Geometry check sheet. Reference: the model listing, model coordinates, mm. A direction names the side the tool comes from. Coordinates: 2 decimals unless noted, no trailing zeros. Loops run counter-clockwise (first coordinate to the right, second up) from the corner with the lowest first, then second, coordinate; pieces in that order, holes last. Notation, with made-up numbers: (86.25, 65) - (90.25, 65) arc R31 cw to (90.25, 102) - close; hole circle Ø6 at (33.25, -32.75). An arc over 180 degrees is marked (long way). Write each question's results on one line, items separated by ' | '. Start each with the question number.
(1) Access from +Z, -Z, +X, -X, +Y, -Y to the whole of each face (thin tool, end or side, straight path). Record for faces 1 (the face through (45, 10, 30)), 2 (the face through (6, 12, 10)), 3 (the face through (31, 9.9, 48.2)), 4 (the face through (30.44, 9.86, 20.76)), 5 (the face through (30, 10, 0)).
(2) Sectioned sample at A-A (z = 31). Enter the section's corners in (x, y), plus the area to 3 significant figures.
(3) Sectioned sample at D-D (y = 18). Enter the section's corners in (x, z).
(4) Sectioned sample at B-B (x = 39). Enter the section's corners in (y, z), plus the area to 3 significant figures.
(5) Material ranges on probe 1 along X at (y, z) = (10, 4); probe 2 along X at (y, z) = (2.75, 41.5); probe 3 along X at (y, z) = (10.5, 3.5) (3 decimals), recorded low to high.
(6) Go/stop test with flat-tipped pins: pin 1 Ø2 at (y, z) = (7, 12) entering from -X; pin 2 Ø5.5 at (x, y) = (7.5, 10) entering from +Z; pin 3 Ø4 at (y, z) = (14.5, 16.5) entering from +X; pin 4 Ø12 at (x, y) = (9.5, 9) entering from +Z. Record where each tip stops, or that it passes through.
(7) Mould release check, pull along Z, two halves, no side actions. Record for faces 6 (the face through (22, 10, 51)), 7 (the face through (30, 0, 19)), 8 (the face through (21.902, 10.585, 43.405)): pulls with the +Z half, pulls with the -Z half, needs draft (parallel to the pull), parting line crosses it, or undercut.
(8) Sectioned sample at C-C (x = 7.5). Enter the section's corners in (y, z), plus the area to 3 significant figures.
from build123d import *

# Parameters (mm, degrees)
BOX002_W                    = 2
BOX002_H                    = 25
BOX002_DEPTH                = 15
CYLINDER003_R               = 2.3
CYLINDER003_DEPTH           = 33
CYLINDER003_PITCH_ANGLE     = 90
CYLINDER003_PLACEMENT_ANGLE = 7e-06
CYLINDER002_R               = 2.3
CYLINDER002_DEPTH           = 13
CYLINDER001_R               = 2.3
CYLINDER001_DEPTH           = 13
CYLINDER_R                  = 10.25
CYLINDER_DEPTH              = 25
CYLINDER_ROLL_ANGLE         = -90
BOX001_W                    = 30
BOX001_H                    = 20
BOX001_DEPTH                = 41
BOX_W                       = 60
BOX_H                       = 20
BOX_DEPTH                   = 10


with BuildPart() as box002:
    # Box002 → Box002 (new body)
    with BuildSketch(Plane(origin=(29, -2.73, 37.37), x_dir=(1, 0, 0), z_dir=(0, 0, 1))):
        with Locations((1, 12.5)):
            Rectangle(BOX002_W, BOX002_H)
    extrude(amount=BOX002_DEPTH)


with BuildPart() as cylinder003:
    # Cylinder003 → Cylinder003 (new body)
    with BuildSketch(Plane.XY):
        Circle(CYLINDER003_R)
    extrude(amount=CYLINDER003_DEPTH)


with BuildPart() as cylinder003_1:
    # Cylinder003 pitch: moved
    add(cylinder003.part.rotate(Axis((0, 0, 0), (0, 1, 0)), CYLINDER003_PITCH_ANGLE))


with BuildPart() as cylinder003_2:
    # Cylinder003 placement: moved
    add(cylinder003_1.part.moved(Location((13.120832, 9.893917, 45.599278))).rotate(Axis((13.120832, 9.893917, 45.599278), (0, 0, 1)), CYLINDER003_PLACEMENT_ANGLE))


with BuildPart() as cylinder002:
    # Cylinder002 → Cylinder002 (new body)
    with BuildSketch(Plane(origin=(52.5, 10, -2), x_dir=(1, 0, 0), z_dir=(0, 0, 1))):
        Circle(CYLINDER002_R)
    extrude(amount=CYLINDER002_DEPTH)


with BuildPart() as cylinder001:
    # Cylinder001 → Cylinder001 (new body)
    with BuildSketch(Plane(origin=(7.5, 10, -2), x_dir=(1, 0, 0), z_dir=(0, 0, 1))):
        Circle(CYLINDER001_R)
    extrude(amount=CYLINDER001_DEPTH)


with BuildPart() as cylinder:
    # Cylinder → Cylinder (new body)
    with BuildSketch(Plane.XY):
        Circle(CYLINDER_R)
    extrude(amount=CYLINDER_DEPTH)


with BuildPart() as cylinder_1:
    # Cylinder roll: moved
    add(cylinder.part.rotate(Axis((0, 0, 0), (1, 0, 0)), CYLINDER_ROLL_ANGLE))


with BuildPart() as cylinder_2:
    # Cylinder placement: moved
    add(cylinder_1.part.moved(Location((30, -3.23131, 31))))


with BuildPart() as cut:
    # Box001 → Box001 (new body)
    with BuildSketch(Plane(origin=(15, 0, 10), x_dir=(1, 0, 0), z_dir=(0, 0, 1))):
        with Locations((15, 10)):
            Rectangle(BOX001_W, BOX001_H)
    extrude(amount=BOX001_DEPTH)

    # Cut: cut Cylinder
    add(cylinder_2.part, mode=Mode.SUBTRACT)


with BuildPart() as cut004:
    # Box → Box (new body)
    with BuildSketch(Plane.XY):
        with Locations((30, 10)):
            Rectangle(BOX_W, BOX_H)
    extrude(amount=BOX_DEPTH)

    # Fusion: union Cut
    add(cut.part)

    # Cut001: cut Cylinder001
    add(cylinder001.part, mode=Mode.SUBTRACT)

    # Cut002: cut Cylinder002
    add(cylinder002.part, mode=Mode.SUBTRACT)

    # Cut003: cut Cylinder003
    add(cylinder003_2.part, mode=Mode.SUBTRACT)

    # Cut004: cut Box002
    add(box002.part, mode=Mode.SUBTRACT)


solid = cut004.part
Outcome:
1) face 1: +Z, +X, +Y, -Y | face 2: +Z, -X, +Y, -Y | face 3: +Z, +Y, -Y | face 4: +Y, -Y | face 5: -Z, +X, -X, +Y, -Y
2) outline: (15, 0) - (19.75, 0) - (19.75, 20) - (15, 20) - close; (40.25, 0) - (45, 0) - (45, 20) - (40.25, 20) - close | area: 190 mm2
3) outline: (0, 0) - (60, 0) - (60, 10) - (45, 10) - (45, 51) - (31, 51) - (31, 41.2) arc R10.25 cw (long way) to (29, 41.2) - (29, 51) - (15, 51) - (15, 10) - (0, 10) - close
4) outline: (0, 0) - (20, 0) - (20, 26.09) - (0, 26.09) - close; (0, 35.91) - (20, 35.91) - (20, 51) - (0, 51) - close; hole circle Ø4.6 at (9.89, 45.6) | area: 807 mm2
5) probe 1: x = 0 to 5.2, 9.8 to 50.2, 54.8 to 60 | probe 2: x = 15 to 29, 31 to 45 | probe 3: x = 0 to 5.255, 9.745 to 50.255, 54.745 to 60
6) pin 1: stops at x = 15 | pin 2: stops at z = 10 | pin 3: stops at x = 45 | pin 4: stops at z = 51
7) face 6: pulls with the +Z half | face 7: needs draft | face 8: undercut
8) outline: (0, 0) - (7.7, 0) - (7.7, 10) - (0, 10) - close; (12.3, 0) - (20, 0) - (20, 10) - (12.3, 10) - close | area: 154 mm2
